Can you work these out from the drawing? Everything is in mm from the part's minimum corner. Give positions to 0.01 mm unless a question says otherwise; leave off trailing zeros. Order: outer loops, then holes, each group sorted by start corner. A loop starts at its lowest first (then second) coordinate and runs counter-clockwise, first axis right, second up. Notation, with made-up numbers: (-39, -36.5) - (-8, -36.5) arc R25 cw to (-8, -11.5) - close; hole circle Ø9 at (79, 55.5). An arc over 180 degrees is marked (long way). Answer as a JSON object with one key per item and string values.
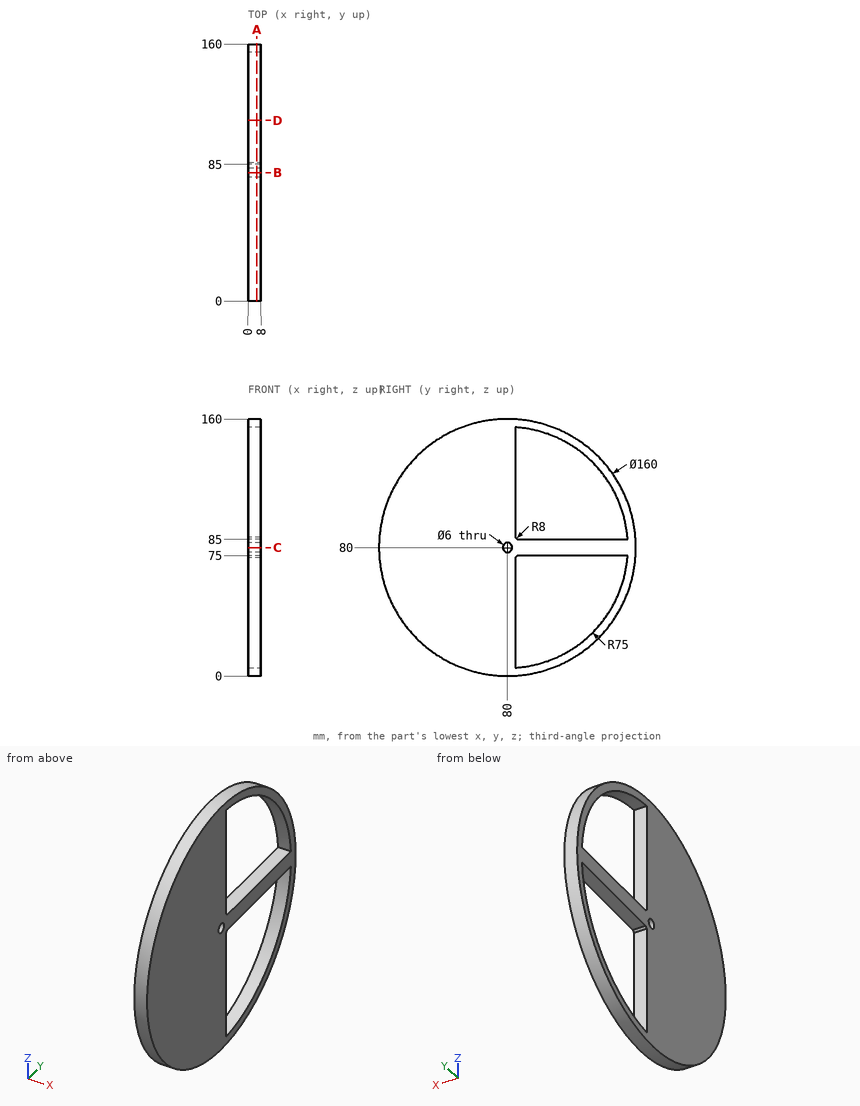
Q1. If we section it at A-A, the plane x = 5.5: Please give me the cut outline in (y, z) (3 decimals), then the cut area to 3 significant figures.
Recorded:
{"outline": "circle Ø160 at (80, 80); hole circle Ø6 at (80, 80); hole (85, 5.167) arc R75 ccw to (154.833, 75) - (86.245, 75) arc R8 cw to (85, 73.755) - close; hole (85, 86.245) arc R8 cw to (86.245, 85) - (154.833, 85) arc R75 ccw to (85, 154.833) - close", "area": "12,700 mm^2"}
Q2. I'm going to push flat-ended pins straight in: pin 1 Ø2.5 at (x, y) = (4, 131.5) entering from +Z; pin 2 Ø4 at (x, z) = (6, 115) entering from +Y; pin 3 Ø1 at (x, z) = (3, 143.5) entering from -Y. Where does each tip first touch, or does it pass through?
Recorded:
{"pin 1": "stops at z = 142.25", "pin 2": "stops at y = 152.88", "pin 3": "stops at y = 30.69"}
Q3. If we section it at D-D, the plane y = 112.5: Please give me the cut outline in (x, z), then the cut area to 3 significant figures.
Recorded:
{"outline": "(0, 6.9) - (8, 6.9) - (8, 12.41) - (0, 12.41) - close; (0, 75) - (8, 75) - (8, 85) - (0, 85) - close; (0, 147.59) - (8, 147.59) - (8, 153.1) - (0, 153.1) - close", "area": "168 mm^2"}
Q4. If we section it at B-B, the plane y = 80: Please give me the cut outline in (x, z), then the cut area to 3 significant figures.
Recorded:
{"outline": "(0, 0) - (8, 0) - (8, 77) - (0, 77) - close; (0, 83) - (8, 83) - (8, 160) - (0, 160) - close", "area": "1,230 mm^2"}
Q5. I need wall thicknesses on L1, parallel to Z at x = 5, y = 80; L2, parallel to Z at x = 4.75, y = 101.5; L3, parallel to Z at x = 1.5, y = 109. Which ranges of each line are inside material? Lowest first, please.
Recorded:
{"L1": "z = 0 to 77, 83 to 160", "L2": "z = 2.94 to 8.15, 75 to 85, 151.85 to 157.06", "L3": "z = 5.44 to 10.83, 75 to 85, 149.17 to 154.56"}
